from build123d import *

# Parameters (mm, degrees)
SKETCH1_R      = 12.5
EXTRUDE1_DEPTH = 7


with BuildPart() as part:
    # Sketch1 → Extrude1 (new body)
    with BuildSketch(Plane(origin=(0, 0, 0), x_dir=(1, 0, 0), z_dir=(0, 1, 0))):
        Polygon((0, 17.320508076), (-15, 8.660254038), (-15, -8.660254038), (0, -17.320508076), (15, -8.660254038), (15, 8.660254038), align=None)
        with Locations(Location((0, 0, 0), (0, 0, 270))):
            Circle(SKETCH1_R, mode=Mode.SUBTRACT)
    extrude(amount=EXTRUDE1_DEPTH)

    # Sketch2 → Cut-Revolve1 (revolve, cut)
    with BuildSketch(Plane(origin=(0, 0, 0), x_dir=(0, 0, -1), z_dir=(1, 0, 0)), mode=Mode.PRIVATE) as cut_revolve1_sk:
        Polygon((0, 4.2), (-16.774097914, 4.2), (-17.120508076, 4.8), (-17.320508076, 4.8), (-17.320508076, 15.108314228), (0, 15.108314228), align=None)
    revolve(cut_revolve1_sk.sketch.rotate(Axis((0, 15.108314228, 0), (0, -1, 0)), 180), axis=Axis((0, 15.108314228, 0), (0, -1, 0)), mode=Mode.SUBTRACT)


solid = part.part
Could you check a few things on this model? Use its own coordinates, in mm. A direction names the side the tool comes from. Round coordinates to 2 decimals unless told otherwise and drop trailing zeros. Write each loop counter-clockwise with the first axis right and the second up, starting at its lowest first coordinate (ties: lowest second). Pieces come first, ordered by that corner, then holes. Notation, with made-up numbers: (76, 58.25) - (90, 58.25) arc R25 cw to (90, 90.25) - close; hole circle Ø2 at (87.5, -28). An arc over 180 degrees is marked (long way). Put each result on its own line as item: value. Start each with the question number.
(1) For faces 1 (the conical face through (-14.653, 4.438, -8.443)), 2 (the flat face through (7.605, 2.366, -12.93)), which set-ups out of +Z, -Z, +X, -X, +Y, -Y let a thin tool reach every point of the face, with its end or its side?
(2) I want a section at C-C, the plane x = -10. Please give me the cut outline in (y, z), plus the area to 3 significant figures.
(3) I want a section at D-D, the plane z = -14. Please give me the cut outline in (x, y).
(4) I want a section at A-A, the plane y = 1.4. Please give me the cut outline in (x, z), plus the area to 3 significant figures.
(5) I want a section at B-B, the plane z = 0. Please give me the cut outline in (x, y).
(6) Will these pins go through, and if not, where does the flat tip stop? pin 1 (8 mm diameter, centred on x = 10.5, z = -2, fed in from +Y); pin 2 (15 mm diameter, centred on x = 3, z = -1, fed in from +Y); pin 3 (12 mm diameter, centred on x = -7, z = 4.5, fed in from -Y).
(7) I need wall thicknesses on probe 1 along Z at (x, y) = (0, 1.95); probe 2 along X at (y, z) = (2.95, 0); probe 3 along Y at (x, z) = (12.5, 8). Which ranges of each line are inside material? Lowest first, please.
(8) Thinking about a two-plate mould opening in Z: for faces 3 (the flat face through (15, 2, 0)), 4 (the conical face through (14.64, 4.44, -8.47)), 5 (the flat face through (1, 4.2, -13)), 6 (the flat face through (-7.4, 1.83, -13.05)), which applies, released by +Z, released by -Z, zero draft, split by the parting line, or undercut?
Here are the results:
1. face 1: +Y
1. face 2: -Z, +X, +Y, -Y
2. outline: (0, -11.55) - (4.2, -11.55) - (4.2, -7.5) - (0, -7.5) - close; (0, 7.5) - (4.2, 7.5) - (4.2, 11.55) - (0, 11.55) - close
2. area: 34.0 mm^2
3. outline: (-5.75, 0) - (5.75, 0) - (5.75, 4.2) - (-5.75, 4.2) - close
4. outline: (-15, -8.66) - (0, -17.32) - (15, -8.66) - (15, 8.66) - (0, 17.32) - (-15, 8.66) - close; hole circle Ø25 at (0, 0)
4. area: 289 mm^2
5. outline: (-15, 0) - (-12.5, 0) - (-12.5, 4.2) - (-15, 4.2) - close; (12.5, 0) - (15, 0) - (15, 4.2) - (12.5, 4.2) - close
6. pin 1: stops at y = 4.2
6. pin 2: passes through
6. pin 3: stops at y = 0
7. probe 1: z = -17.32 to -12.5, 12.5 to 17.32
7. probe 2: x = -15 to -12.5, 12.5 to 15
7. probe 3: y = 0 to 4.2
8. face 3: zero draft
8. face 4: undercut
8. face 5: undercut
8. face 6: released by -Z
